The drawing under review shows one solid part. Ordinate dimensions are in mm from its lowest x, y, z. A direction names the side the tool comes from. Give positions to 0.01 mm unless a question says otherwise; leave off trailing zeros. Loops run counter-clockwise (first coordinate to the right, second up) from the corner with the lowest first, then second, coordinate; pieces in that order, holes last. Notation, with made-up numbers: M 58.5,-14.5 L 84.5,-14.5 A19 ccw 84.5,7.5 Z; hole C -27,-13 d9. An arc over 180 degrees is marked long. One line per item, written item: value. Start each with the question number.
Q1. We need section B-B on z = 40. Write out the cut boundary in (x, y), plus the area to 3 significant figures.
Q2. We need section C-C on y = 115. Write out the cut boundary in (x, z).
Q3. For the marked faces 1 and 2, list the 3-axis set-ups (+Z, -Z, +X, -X, +Y, -Y) from which the entire face can be reached by the end or side of a thin tool; tool diameter is ignored.
Q4. We need section D-D on z = 16.5. Write out the cut boundary in (x, y), plus the area to 3 significant figures.
Q5. We need section A-A on x = 40. Write out the cut boundary in (y, z), plus the area to 3 significant figures.
Q6. For pin 1 (1.5 mm diameter, centred on y = 65.5, z = 69.5, fed in from -X), flat-tipped, find the tip position at first contact; note if it passes through.
Q7. To check wall thickness, follow line 1 along Z through (x, y) = (40, 2.45); line 2 along Y through (x, z) = (121.3, 40); line 3 along Y through (x, z) = (21, 70). State the ranges of each line that lie inside material, in increasing order. Write a range as from..to.
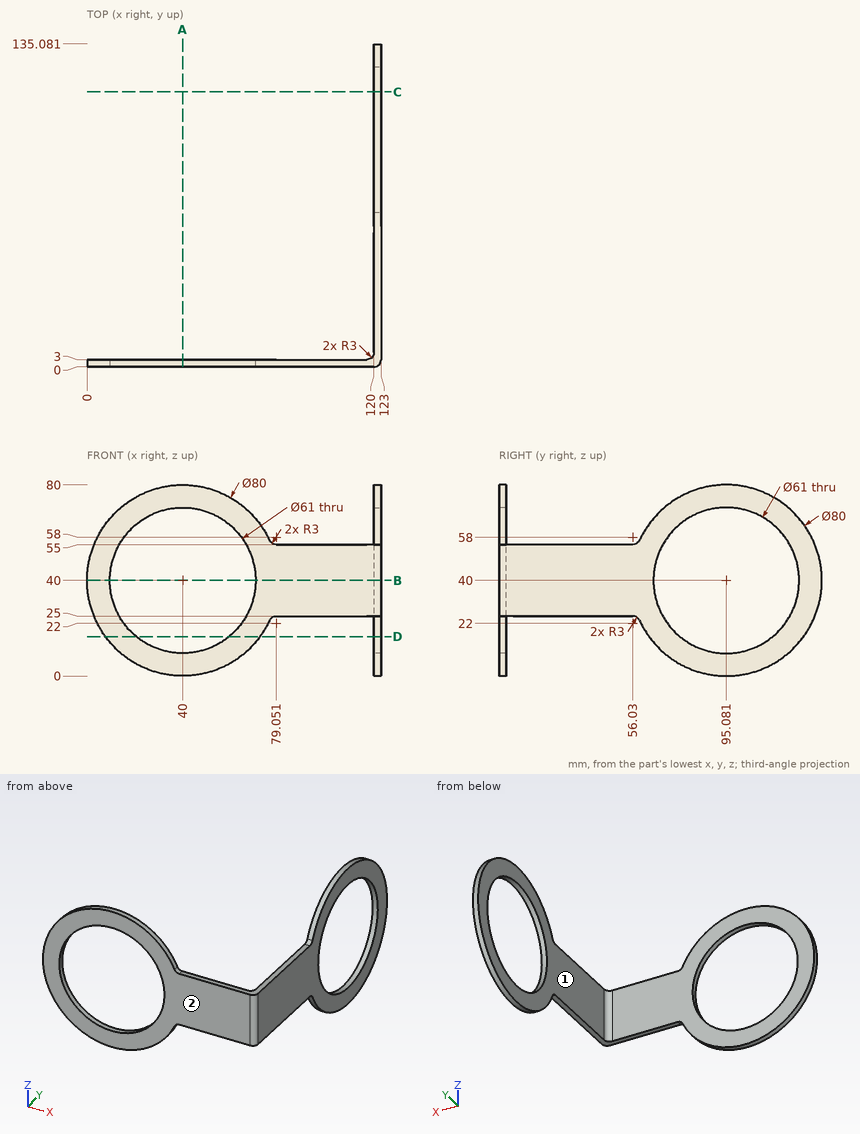
Solved:
1. outline: M 0,0 L 9.5,0 L 9.5,3 L 0,3 Z; M 70.5,0 L 120,0 A3 ccw 123,3 L 123,64.58 L 120,64.58 L 120,6 A3 cw 117,3 L 70.5,3 Z; M 120,125.58 L 123,125.58 L 123,135.08 L 120,135.08 Z
1. area: 399 mm2
2. outline: M 120,5.31 L 123,5.31 L 123,16.9 L 120,16.9 Z; M 120,63.1 L 123,63.1 L 123,74.69 L 120,74.69 Z
3. face 1: +Z, -Z, -X, +Y
3. face 2: +Z, -Z, +X, -X, -Y
4. outline: M 7.63,0 L 20.56,0 L 20.56,3 L 7.63,3 Z; M 59.44,0 L 72.37,0 L 72.37,3 L 59.44,3 Z; M 120,62.71 L 123,62.71 L 123,75.64 L 120,75.64 Z; M 120,114.52 L 123,114.52 L 123,127.45 L 120,127.45 Z
4. area: 155 mm2
5. outline: M 0,0 L 3,0 L 3,9.5 L 0,9.5 Z; M 0,70.5 L 3,70.5 L 3,80 L 0,80 Z
5. area: 57.0 mm2
6. pin 1: through
7. line 1: 0..9.5, 70.5..80
7. line 2: 0.3..64.58, 125.58..135.08
7. line 3: 0..3
